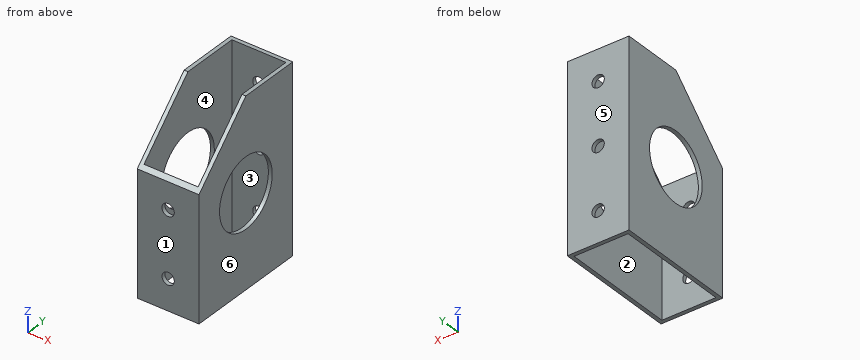
from build123d import *

# Parameters (mm, degrees)
SKETCH1_W           = 25.4
SKETCH1_H           = 50.8
SKETCH1_W_2         = 22.225
SKETCH1_H_2         = 47.625
BOSS_EXTRUDE1_DEPTH = 76.2
SKETCH2_R           = 14.2875
CUT_EXTRUDE1_DEPTH  = 96.038097624
CUT_EXTRUDE2_DEPTH  = 96.038097624
CUT_EXTRUDE3_REACH  = 97.038
SKETCH4_R           = 2.54
CUT_EXTRUDE4_REACH  = 97.038
SKETCH5_R           = 2.54


with BuildPart() as part:
    # Sketch1 → Boss-Extrude1 (new body)
    with BuildSketch(Plane.XY):
        with Locations((12.7, 25.4)):
            Rectangle(SKETCH1_W, SKETCH1_H)
        with Locations((12.7, 25.4)):
            Rectangle(SKETCH1_W_2, SKETCH1_H_2, mode=Mode.SUBTRACT)
    extrude(amount=BOSS_EXTRUDE1_DEPTH)

    # Sketch2 → Cut-Extrude1 (cut, through all)
    with BuildSketch(Plane(origin=(25.4, 0, 0), x_dir=(0, 0, -1), z_dir=(1, 0, 0))):
        with Locations((-38.1, 25.4)):
            Circle(SKETCH2_R)
    extrude(amount=-CUT_EXTRUDE1_DEPTH, mode=Mode.SUBTRACT)

    # Sketch3 → Cut-Extrude2 (cut, through all)
    with BuildSketch(Plane(origin=(25.4, 0, 0), x_dir=(0, 0, -1), z_dir=(1, 0, 0))):
        Polygon((-50.8, 0), (-76.2, 25.4), (-76.2, 0), align=None)
    extrude(amount=-CUT_EXTRUDE2_DEPTH, mode=Mode.SUBTRACT)

    # Sketch4 → Cut-Extrude3 (cut, up to next)
    with BuildSketch(Plane(origin=(0, 50.8, 0), x_dir=(1, 0, 0), z_dir=(0, 1, 0)), mode=Mode.PRIVATE) as cut_extrude3_sk1:
        with Locations(Location((12.7, -12.7, 0), (0, 0, 270))):
            Circle(SKETCH4_R)
    cut_extrude3_tool1 = extrude(cut_extrude3_sk1.sketch, amount=-CUT_EXTRUDE3_REACH, mode=Mode.PRIVATE) & part.part
    # Sketch4 → Cut-Extrude3 (cut, up to next)
    with BuildSketch(Plane(origin=(0, 50.8, 0), x_dir=(1, 0, 0), z_dir=(0, 1, 0)), mode=Mode.PRIVATE) as cut_extrude3_sk2:
        with Locations(Location((12.7, -38.1, 0), (0, 0, 270))):
            Circle(SKETCH4_R)
    cut_extrude3_tool2 = extrude(cut_extrude3_sk2.sketch, amount=-CUT_EXTRUDE3_REACH, mode=Mode.PRIVATE) & part.part
    # Sketch4 → Cut-Extrude3 (cut, up to next)
    with BuildSketch(Plane(origin=(0, 50.8, 0), x_dir=(1, 0, 0), z_dir=(0, 1, 0)), mode=Mode.PRIVATE) as cut_extrude3_sk3:
        with Locations(Location((12.7, -63.5, 0), (0, 0, 270))):
            Circle(SKETCH4_R)
    cut_extrude3_tool3 = extrude(cut_extrude3_sk3.sketch, amount=-CUT_EXTRUDE3_REACH, mode=Mode.PRIVATE) & part.part
    add(cut_extrude3_tool1.solids().sort_by_distance((12.7, 50.8, 12.7))[0], mode=Mode.SUBTRACT)
    add(cut_extrude3_tool2.solids().sort_by_distance((12.7, 50.8, 38.1))[0], mode=Mode.SUBTRACT)
    add(cut_extrude3_tool3.solids().sort_by_distance((12.7, 50.8, 63.5))[0], mode=Mode.SUBTRACT)

    # Sketch5 → Cut-Extrude4 (cut, up to next)
    with BuildSketch(Plane.XZ, mode=Mode.PRIVATE) as cut_extrude4_sk1:
        with Locations(Location((12.7, 12.7, 0), (0, 0, 90))):
            Circle(SKETCH5_R)
    cut_extrude4_tool1 = extrude(cut_extrude4_sk1.sketch, amount=-CUT_EXTRUDE4_REACH, mode=Mode.PRIVATE) & part.part
    # Sketch5 → Cut-Extrude4 (cut, up to next)
    with BuildSketch(Plane.XZ, mode=Mode.PRIVATE) as cut_extrude4_sk2:
        with Locations(Location((12.7, 39.6875, 0), (0, 0, 270))):
            Circle(SKETCH5_R)
    cut_extrude4_tool2 = extrude(cut_extrude4_sk2.sketch, amount=-CUT_EXTRUDE4_REACH, mode=Mode.PRIVATE) & part.part
    add(cut_extrude4_tool1.solids().sort_by_distance((12.7, 0, 12.7))[0], mode=Mode.SUBTRACT)
    add(cut_extrude4_tool2.solids().sort_by_distance((12.7, 0, 39.6875))[0], mode=Mode.SUBTRACT)


solid = part.part
Can you work these out from the model? Positions are in its coordinate system, mm. Face numbers are marked on the shaded views. A direction names the side the tool comes from. Coordinates: 2 decimals unless noted, no trailing zeros. Order: outer loops, then holes, each group sorted by start corner. A loop starts at its lowest first (then second) coordinate and runs counter-clockwise, first axis right, second up. Notation, with made-up numbers: M 2,-26 L 61,-26 A24 ccw 61,3 Z; hole C 36,19.5 d3. An arc over 180 degrees is marked long. Answer as CSV lines item,"result".
(1) If we mould it in two halves opening along X, with no side actions, what happens to the marked faces 3, 4, 5 and 6? For each: released by +X, released by -X, zero draft, split by the parting line, or undercut.
Geometry check:
face 3,"undercut"
face 4,"undercut"
face 5,"zero draft"
face 6,"released by +X"
(2) Suppose I cut it at D-D on z = 23. Please give me the cut outline in (x, y), plus the area to 3 significant figures.
Geometry check:
outline,"M 0,0 L 25.4,0 L 25.4,50.8 L 0,50.8 Z; hole M 1.59,1.59 L 23.81,1.59 L 23.81,49.21 L 1.59,49.21 Z"
area,"232 mm^2"
(3) Suppose I cut it at A-A on z = 63.5. Please give me the cut outline in (x, y).
Geometry check:
outline,"M 0,12.7 L 1.59,12.7 L 1.59,49.21 L 10.16,49.21 L 10.16,50.8 L 0,50.8 Z; M 15.24,49.21 L 23.81,49.21 L 23.81,12.7 L 25.4,12.7 L 25.4,50.8 L 15.24,50.8 Z"
(4) On a 3-axis mill with a long thin cutter (end or side, diameter ignored), from which of +Z, -Z, +X, -X, +Y, -Y can I reach the whole of each face in a straight line? I mean the marked faces 1 and 2. Say none if no direction works.
Geometry check:
face 1,"+Z, -Z, +X, -X, -Y"
face 2,"+Z, -Z"
(5) Suppose I cut it at B-B on x = 7.25. Please give me the cut outline in (y, z), plus the area to 3 significant figures.
Geometry check:
outline,"M 0,0 L 1.59,0 L 1.59,52.39 L 0,50.8 Z; M 49.21,0 L 50.8,0 L 50.8,76.2 L 49.21,76.2 Z"
area,"203 mm^2"
(6) Please list where these lines run through material, in increasing order: L1, parallel to Y at x = 10, z = 22.5; L2, parallel to X at y = 18.5, z = 8; L3, parallel to X at y = 50.1, z = 38.1.
Geometry check:
L1,"0 to 1.59, 49.21 to 50.8"
L2,"0 to 1.59, 23.81 to 25.4"
L3,"0 to 10.16, 15.24 to 25.4"
(7) I'm going to push flat-ended pins straight in: pin 1 (3 mm diameter, centred on x = 12.7, z = 12.7, fed in from +Y); pin 2 (4 mm diameter, centred on x = 12.7, z = 39.69, fed in from -Y). Where does each tip first touch, or does it pass through?
Geometry check:
pin 1,"through"
pin 2,"y = 49.21"
(8) Suppose I cut it at C-C on y = 42. Please give me the cut outline in (x, z).
Geometry check:
outline,"M 0,0 L 1.59,0 L 1.59,76.2 L 0,76.2 Z; M 23.81,0 L 25.4,0 L 25.4,76.2 L 23.81,76.2 Z"
